Could you check a few things on this model? Use its own coordinates, in mm. Face numbers are marked on the shaded views. A direction names the side the tool comes from. Coordinates: 2 decimals unless noted, no trailing zeros. Loops run counter-clockwise (first coordinate to the right, second up) from the corner with the lowest first, then second, coordinate; pieces in that order, holes last. Notation, with made-up numbers: M -32.5,0 L -21.5,0 A25 ccw -21.5,33 Z; hole C 1.5,0 d8. An arc over 180 degrees is marked long. Write each question's results on one line, items separated by ' | '.
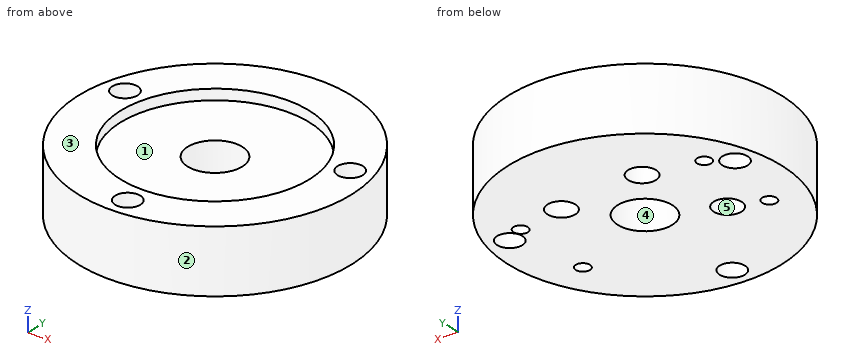
```python
from build123d import *

# Parameters (mm, degrees)
ESQUISSE1_R                = 32.5
BOSS_EXTRU_1_DEPTH         = 15
ESQUISSE2_R                = 22.5
ENL_V_MAT_EXTRU_1_DEPTH    = 2.5
ESQUISSE3_R                = 6.5
ENL_V_MAT_EXTRU_2_DEPTH    = 48.631397208
TROUS_DE_CENTRAGE_6_0MM1_D = 6
D_GAGEMENT_M61_D           = 6.6
D_GAGEMENT_M61_DEPTH       = 5
D_GAGEMENT_M61_TIP         = 1.905255888
D_GAGEMENT_M31_D           = 3.4
D_GAGEMENT_M31_DEPTH       = 5
D_GAGEMENT_M31_TIP         = 0.981495458
D_GAGEMENT_M32_D           = 3.4
D_GAGEMENT_M32_DEPTH       = 5
D_GAGEMENT_M32_TIP         = 0.981495458


with BuildPart() as part:
    # Esquisse1 → Boss.-Extru.1 (new body)
    with BuildSketch(Plane.XY):
        Circle(ESQUISSE1_R)
    extrude(amount=BOSS_EXTRU_1_DEPTH)

    # Esquisse2 → Enlèv. mat.-Extru.1 (cut)
    with BuildSketch(Plane.XY.offset(15)):
        Circle(ESQUISSE2_R)
    extrude(amount=-ENL_V_MAT_EXTRU_1_DEPTH, mode=Mode.SUBTRACT)

    # Esquisse3 → Enlèv. mat.-Extru.2 (cut, through all)
    with BuildSketch(Plane.XY.offset(12.5)):
        Circle(ESQUISSE3_R)
    extrude(amount=-ENL_V_MAT_EXTRU_2_DEPTH, mode=Mode.SUBTRACT)

    # Trous de centrage Ø6.0mm1 (through all)
    with Locations(Plane.XY.offset(15)):
        with Locations((0, -27.5), (-26.562960223, 7.11752374), (26.562960223, 7.11752374)):
            Hole(TROUS_DE_CENTRAGE_6_0MM1_D / 2)

    # Dégagement M61
    with Locations(Plane(origin=(0, 0, 0), x_dir=(-1, 0, 0), z_dir=(0, 0, -1))):
        with Locations((-11.303753991, 11.241031035), (9.107378233, 13.084009123), (14.466713258, -6.697002353)):
            Hole(D_GAGEMENT_M61_D / 2, depth=D_GAGEMENT_M61_DEPTH)
            with Locations((0, 0, -(D_GAGEMENT_M61_DEPTH + D_GAGEMENT_M61_TIP / 2))):  # 120° drill point
                Cone(0, D_GAGEMENT_M61_D / 2, D_GAGEMENT_M61_TIP, mode=Mode.SUBTRACT)

    # Dégagement M31
    with Locations(Plane(origin=(0, 0, 0), x_dir=(-1, 0, 0), z_dir=(0, 0, -1))):
        with Locations((22.298556593, -9.388080653), (21.906177888, 10.608069951)):
            Hole(D_GAGEMENT_M31_D / 2, depth=D_GAGEMENT_M31_DEPTH)
            with Locations((0, 0, -(D_GAGEMENT_M31_DEPTH + D_GAGEMENT_M31_TIP / 2))):  # 120° drill point
                Cone(0, D_GAGEMENT_M31_D / 2, D_GAGEMENT_M31_TIP, mode=Mode.SUBTRACT)

    # Dégagement M32
    with Locations(Plane(origin=(0, 0, 0), x_dir=(-1, 0, 0), z_dir=(0, 0, -1))):
        with Locations((-21.92383493, -9.708243173), (-22.298556593, 9.388080653)):
            Hole(D_GAGEMENT_M32_D / 2, depth=D_GAGEMENT_M32_DEPTH)
            with Locations((0, 0, -(D_GAGEMENT_M32_DEPTH + D_GAGEMENT_M32_TIP / 2))):  # 120° drill point
                Cone(0, D_GAGEMENT_M32_D / 2, D_GAGEMENT_M32_TIP, mode=Mode.SUBTRACT)


solid = part.part
```
(1) Please list where these lines run through material, in increasing order: probe 1 along Y at (x, z) = (0, 8.5); probe 2 along Y at (x, z) = (-21, 1); probe 3 along X at (y, z) = (7.5, 8.75). Write a range as from..to.
Reported:
probe 1: y = -32.5..-30.5, -24.5..-6.5, 6.5..32.5 | probe 2: y = -24.8..-10.49, -8.29..9.17, 12.05..24.8 | probe 3: x = -31.62..-29.54, -23.59..23.59, 29.54..31.62
(2) Imagine slicing it at B-B, the plane x = 0. List the corners of the cut face in (y, z) for me.
Reported:
outline: M -32.5,0 L -30.5,0 L -30.5,15 L -32.5,15 Z; M -24.5,0 L -6.5,0 L -6.5,12.5 L -22.5,12.5 L -22.5,15 L -24.5,15 Z; M 6.5,0 L 32.5,0 L 32.5,15 L 22.5,15 L 22.5,12.5 L 6.5,12.5 Z
(3) Imagine slicing it at C-C, the plane z = 3.25. State how many separate pieces and enclosed holes the cut face has, and give its area (3 significant figures).
Reported:
separate pieces: 1 | enclosed holes: 11 | area: 2,960 mm2
(4) Imagine slicing it at A-A, the plane y = 0. List the corners of the cut face in (x, z) for me, and give its area (3 significant figures).
Reported:
outline: M -32.5,0 L -6.5,0 L -6.5,12.5 L -22.5,12.5 L -22.5,15 L -32.5,15 Z; M 6.5,0 L 32.5,0 L 32.5,15 L 22.5,15 L 22.5,12.5 L 6.5,12.5 Z | area: 700 mm2
(5) If we mould it in two halves opening along X, with no side actions, what happens to the marked faces 1, 2 and 3? For each: released by +X, released by -X, zero draft, split by the parting line, or undercut.
Reported:
face 1: undercut | face 2: split by the parting line | face 3: zero draft
(6) Will these pins go through, and if not, where does the flat tip stop? P1, Ø1.5, axis at x = 12.5, y = 6.5, coming from the +Z side; P2, Ø5, axis at x = 0, y = -27.5, coming from the -Z side; P3, Ø6, axis at x = 11.3, y = 11.24, coming from the -Z side; P4, Ø2, axis at x = -21.91, y = 10.61, coming from the -Z side.
Reported:
P1: stops at z = 12.5 | P2: passes through | P3: stops at z = 5.17 | P4: stops at z = 5.4
(7) Imagine slicing it at D-D, the plane x = 16.5. List the corners of the cut face in (y, z) for me, and give its area (3 significant figures).
Reported:
outline: M -28,0 L 28,0 L 28,15 L 15.3,15 L 15.3,12.5 L -15.3,12.5 L -15.3,15 L -28,15 Z | area: 764 mm2
(8) Which directions (+Z, -Z, +X, -X, +Y, -Y) give clear straight access to the entire face, cutting with the end or side of a thin tool? Please do the marked faces 4 and 5.
Reported:
face 4: +Z, -Z | face 5: -Z
